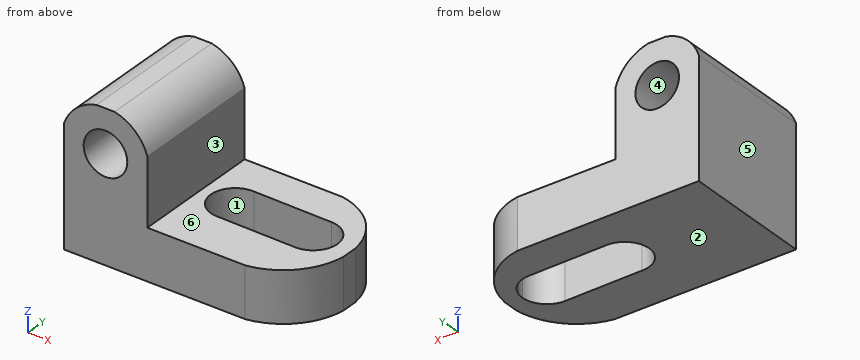
from build123d import *

# Parameters (mm, degrees)
F1_DEPTH = 25.4
F3_DEPTH = 9.7799997235
F5_DEPTH = 9.7799997235
F7_DEPTH = 25.401
F8_R     = 4.2081540675
F9_DEPTH = 25.401


with BuildPart() as f1:
    # F0 (on Front) → F1 (new body)
    with BuildSketch(Plane.XZ):
        Polygon((0, 28.5467784852), (0, 0), (45.7341149449, 0), (45.7341149449, 9.7789997235), (16.1007773131, 9.7789997235), (16.1007773131, 28.5467784852), align=None)
    extrude(amount=F1_DEPTH)

    # F2 (on face) → F3 (cut, through all)
    with BuildSketch(Plane.XY.offset(9.7789997235)):
        with BuildLine():
            ThreePointArc((23.013047613, -16.2487795257), (26.2065060315, -14.8076541333), (27.5135145448, -11.5570006892))
            ThreePointArc((27.5135145448, -11.5570006892), (26.2065060315, -8.3063472451), (23.013047613, -6.8652218527))
            ThreePointArc((23.013047613, -6.8652218527), (18.1218243279, -11.5570006892), (23.013047613, -16.2487795257))
        make_face()
        with BuildLine():
            ThreePointArc((23.013047613, -6.8652218527), (26.2065060315, -8.3063472451), (27.5135145448, -11.5570006892))
            ThreePointArc((27.5135145448, -11.5570006892), (26.2065060315, -14.8076541333), (23.013047613, -16.2487795257))
            Line((23.013047613, -16.2487795257), (37.966271611, -16.4499710275))
            ThreePointArc((37.966271611, -16.4499710275), (33.334012479, -11.6927764727), (38.0898284635, -7.0591020107))
            Line((38.0898284635, -7.0591020107), (23.013047613, -6.8652218527))
        make_face()
        with BuildLine():
            ThreePointArc((42.7252883073, -11.7545549017), (41.3711881032, -8.4555108805), (38.0898284635, -7.0591020107))
            ThreePointArc((38.0898284635, -7.0591020107), (33.334012479, -11.6927764727), (37.966271611, -16.4499710275))
            ThreePointArc((37.966271611, -16.4499710275), (41.327496713, -15.0972773142), (42.7252883073, -11.7545549017))
        make_face()
    extrude(amount=-F3_DEPTH, mode=Mode.SUBTRACT)

    # F4 (on face) → F5 (cut, through all)
    with BuildSketch(Plane.XY.offset(9.7789997235)):
        with BuildLine():
            ThreePointArc((35.0055416845, 0), (42.2404327965, -3.7910480752), (45.7341149449, -11.17412873))
            Line((45.7341149449, -11.17412873), (45.7341149449, 0))
            Line((45.7341149449, 0), (35.0055416845, 0))
        make_face()
        with BuildLine():
            ThreePointArc((45.7341149449, -14.22587127), (42.2404327965, -21.6089519248), (35.0055416845, -25.4))
            Line((35.0055416845, -25.4), (45.7341149449, -25.4))
            Line((45.7341149449, -25.4), (45.7341149449, -14.22587127))
        make_face()
    extrude(amount=-F5_DEPTH, mode=Mode.SUBTRACT)

    # F6 (on face) → F7 (cut, through all)
    with BuildSketch(Plane.XZ.offset(25.4)):
        with BuildLine():
            ThreePointArc((0, 22.8922715803), (2.3876784288, 26.566481818), (6.2965470963, 28.5467784852))
            Line((6.2965470963, 28.5467784852), (0, 28.5467784852))
            Line((0, 28.5467784852), (0, 22.8922715803))
        make_face()
        with BuildLine():
            ThreePointArc((9.7487572031, 28.5467784852), (13.7265705753, 26.5038761141), (16.1007773131, 22.7144709249))
            Line((16.1007773131, 22.7144709249), (16.1007773131, 28.5467784852))
            Line((16.1007773131, 28.5467784852), (9.7487572031, 28.5467784852))
        make_face()
    extrude(amount=-F7_DEPTH, mode=Mode.SUBTRACT)

    # F8 (on face) → F9 (cut, through all)
    with BuildSketch(Plane.XZ.offset(25.4)):
        with Locations((8.0226521497, 20.2916857982)):
            Circle(F8_R)
    extrude(amount=-F9_DEPTH, mode=Mode.SUBTRACT)


solid = f1.part
For this review, take the finished solid that the model builds, in its own axes (mm). Face numbers are marked on the shaded views. A direction names the side the tool comes from. Round coordinates to 2 decimals unless told otherwise and drop trailing zeros. Loops run counter-clockwise (first coordinate to the right, second up) from the corner with the lowest first, then second, coordinate; pieces in that order, holes last. Notation, with made-up numbers: (-30, -15.75) - (-1, -15.75) arc R15 cw to (-1, 10.25) - close; hole circle Ø11 at (49, 34.5). An arc over 180 degrees is marked (long way). Put each result on its own line as item: value. Start each with the question number.
1. For probe 1 along X at (y, z) = (-6, 20.25); probe 2 along Y at (x, z) = (23, 8); probe 3 along Z at (x, y) = (40, -19.5), list the stretches that pass through material, from the lowest coordinate up. Write a range as [from, to].
2. Consider section D-D on z = 18.75. State the section outline as (x, y) points.
3. Mouldability with a two-part tool opening along X and no side actions: class the marked faces 4, 5 and 6 as +X half, -X half, draft (parallel to the pull), parting line (faces both ways), or undercut.
4. For the marked faces 1, 2 and 3, list the 3-axis set-ups (+Z, -Z, +X, -X, +Y, -Y) from which the entire face can be reached by the end or side of a thin tool; tool diameter is ignored.
5. Consider section C-C on x = 8.5. State the section outline as (y, z) points, plus the area to 3 significant figures.
6. Consider section B-B on y = -12.5. State the section outline as (x, z) points.
7. Insertion check: P1, Ø1.5, axis at y = -9.5, z = 4.5, coming from the +X side; P2, Ø4, axis at y = -13, z = 20.5, coming from the +X side; P3, Ø4, axis at y = -21, z = 4, coming from the +X side. Each pin has a flat end and moves straight along its axis. Give the tip position at first contact, or say it passes through.
8. Consider section A-A on z = 9. State the section outline as (x, y) points.
Result sheet:
1. probe 1: [0, 3.81], [12.23, 16.1]
1. probe 2: [-25.4, -16.25], [-6.86, 0]
1. probe 3: [0, 9.78]
2. outline: (0, -25.4) - (4.11, -25.4) - (4.11, 0) - (0, 0) - close; (11.94, -25.4) - (16.1, -25.4) - (16.1, 0) - (11.94, 0) - close
3. face 4: undercut
3. face 5: -X half
3. face 6: draft
4. face 1: +Z, -Z
4. face 2: -Z, +X, -X, +Y, -Y
4. face 3: +Z, +X, +Y, -Y
5. outline: (-25.4, 0) - (0, 0) - (0, 16.11) - (-25.4, 16.11) - close; (-25.4, 24.47) - (0, 24.47) - (0, 28.55) - (-25.4, 28.55) - close
5. area: 513 mm^2
6. outline: (0, 0) - (18.22, 0) - (18.22, 9.78) - (16.1, 9.78) - (16.1, 22.71) arc R8.43 ccw to (9.75, 28.55) - (6.3, 28.55) arc R8.43 ccw to (0, 22.89) - close; (42.67, 0) - (45.73, 0) - (45.73, 9.78) - (42.67, 9.78) - close; hole circle Ø8.42 at (8.02, 20.29)
7. P1: x = 45.59
7. P2: x = 16.1
7. P3: x = 44.18
8. outline: (0, -25.4) - (35.01, -25.4) arc R12.86 ccw to (45.73, -14.23) - (45.73, -11.17) arc R12.86 ccw to (35.01, 0) - (0, 0) - close; hole (23.01, -16.25) - (37.97, -16.45) arc R4.7 ccw to (38.09, -7.06) - (23.01, -6.87) arc R4.7 ccw (long way) to start
